from build123d import *

# Parameters (mm, degrees)
SKIZZE1_W                       = 155
SKIZZE1_H                       = 23
SKIZZE1_W_2                     = 147
SKIZZE1_H_2                     = 15
AUFSATZ_LINEAR_AUSTRAGEN1_DEPTH = 10
SKIZZE3_W                       = 155
SKIZZE3_H                       = 23
AUFSATZ_LINEAR_AUSTRAGEN3_DEPTH = 4
SKIZZE4_W                       = 149
SKIZZE4_H                       = 17
SKIZZE4_W_2                     = 147
SKIZZE4_H_2                     = 15
SCHNITT_LINEAR_AUSTRAGEN1_DEPTH = 0.5
SKIZZE5_W                       = 149
SKIZZE5_H                       = 17
SCHNITT_LINEAR_AUSTRAGEN2_DEPTH = 0.5


with BuildPart() as part:
    # Skizze1 → Aufsatz-Linear austragen1 (new body)
    with BuildSketch(Plane(origin=(0, 0, 0), x_dir=(1, 0, 0), z_dir=(0, 1, 0))):
        Rectangle(SKIZZE1_W, SKIZZE1_H)
        Rectangle(SKIZZE1_W_2, SKIZZE1_H_2, mode=Mode.SUBTRACT)
    extrude(amount=AUFSATZ_LINEAR_AUSTRAGEN1_DEPTH)

    # Skizze3 → Aufsatz-Linear austragen3 (add)
    with BuildSketch(Plane.XZ):
        Rectangle(SKIZZE3_W, SKIZZE3_H)
    extrude(amount=AUFSATZ_LINEAR_AUSTRAGEN3_DEPTH)

    # Skizze4 → Schnitt-Linear austragen1 (cut)
    with BuildSketch(Plane(origin=(0, 4, 0), x_dir=(1, 0, 0), z_dir=(0, 1, 0))):
        Rectangle(SKIZZE4_W, SKIZZE4_H)
        Rectangle(SKIZZE4_W_2, SKIZZE4_H_2, mode=Mode.SUBTRACT)
    extrude(amount=SCHNITT_LINEAR_AUSTRAGEN1_DEPTH, mode=Mode.SUBTRACT)

    # Skizze5 → Schnitt-Linear austragen2 (cut)
    with BuildSketch(Plane(origin=(0, 6, 0), x_dir=(1, 0, 0), z_dir=(0, 1, 0))):
        Rectangle(SKIZZE5_W, SKIZZE5_H)
    extrude(amount=SCHNITT_LINEAR_AUSTRAGEN2_DEPTH, mode=Mode.SUBTRACT)


solid = part.part
Read the model definition and answer for the solid it produces. Units are mm, in the model's axes. A direction names the side the tool comes from. Coordinates: 2 decimals unless noted, no trailing zeros. Order: outer loops, then holes, each group sorted by start corner. A loop starts at its lowest first (then second) coordinate and runs counter-clockwise, first axis right, second up. Notation, with made-up numbers: M 66.5,11 L 96.5,11 A30 cw 96.5,44 Z; hole C -31.75,26 d6. An arc over 180 degrees is marked long. Put each result on its own line as item: value. Start each with the question number.
Item 1: The mould has two halves that part along Y. Classify faces 1 (the face through (73.5, 8, 0)), 2 (the face through (-1, 0, 0)), 3 (the face through (0, 6.5, -8)), 4 (the face through (0, 4.5, -8)): +Y half, -Y half, draft (parallel to the pull), parting line (faces both ways), or undercut.
Item 2: For faces 5 (the face through (0, 6, -8)), 6 (the face through (77.5, 3, 0)), 7 (the face through (-73.5, 8, 0)), determine the directions among +Z, -Z, +X, -X, +Y, -Y from which every point of the face is accessible in a straight line to the end or side of a thin tool.
Item 3: Section B-B, the plane z = -4 is taken. Determine the outline of the cut face in (x, y).
Item 4: Section A-A, the plane y = 2 is taken. Determine the outline of the cut face in (x, z), plus the area to 3 significant figures.
Item 5: Section C-C, the plane x = -60.5 is taken. Determine the outline of the cut face in (y, z).
Item 6: Consider probe 1 along Y at (x, z) = (-40.5, -8.25); probe 2 along Z at (x, y) = (3.5, 7.25); probe 3 along X at (y, z) = (7.5, -2.75). Determine where each line is inside the solid, lowest interval first. Write a range as [from, to].
Computed:
1. face 1: draft
1. face 2: +Y half
1. face 3: undercut
1. face 4: undercut
2. face 5: none
2. face 6: +Z, -Z, +X, +Y, -Y
2. face 7: +Y
3. outline: M -77.5,-4 L 77.5,-4 L 77.5,10 L 73.5,10 L 73.5,6.5 L 74.5,6.5 L 74.5,6 L 73.5,6 L 73.5,4.5 L 74.5,4.5 L 74.5,4 L 73.5,4 L 73.5,0 L -73.5,0 L -73.5,4 L -74.5,4 L -74.5,4.5 L -73.5,4.5 L -73.5,6 L -74.5,6 L -74.5,6.5 L -73.5,6.5 L -73.5,10 L -77.5,10 Z
4. outline: M -77.5,-11.5 L 77.5,-11.5 L 77.5,11.5 L -77.5,11.5 Z; hole M -73.5,-7.5 L 73.5,-7.5 L 73.5,7.5 L -73.5,7.5 Z
4. area: 1,360 mm2
5. outline: M -4,-11.5 L 10,-11.5 L 10,-7.5 L 6.5,-7.5 L 6.5,-8.5 L 6,-8.5 L 6,-7.5 L 4.5,-7.5 L 4.5,-8.5 L 4,-8.5 L 4,-7.5 L 0,-7.5 L 0,7.5 L 4,7.5 L 4,8.5 L 4.5,8.5 L 4.5,7.5 L 6,7.5 L 6,8.5 L 6.5,8.5 L 6.5,7.5 L 10,7.5 L 10,11.5 L -4,11.5 Z
6. probe 1: y = [-4, 4], [4.5, 6], [6.5, 10]
6. probe 2: z = [-11.5, -7.5], [7.5, 11.5]
6. probe 3: x = [-77.5, -73.5], [73.5, 77.5]
